Part model, mm, in its own coordinate system. Face numbers are marked on the shaded views. A direction names the side the tool comes from. Give positions to 0.01 mm unless a question says otherwise; leave off trailing zeros. Order: outer loops, then holes, each group sorted by start corner. A loop starts at its lowest first (then second) coordinate and runs counter-clockwise, first axis right, second up.
1. Slice it at D-D on z = 36. List the corners of the cut face in (x, y), and give its area (3 significant figures).
2. Which spindle directions (+Z, -Z, +X, -X, +Y, -Y) get a long thin tool onto all of the face, cutting with end or side? Do the marked faces 1 and 2. Say none if no direction does.
3. Slice it at B-B on y = 0. List the corners of the cut face in (x, z).
4. Probe line 1 (Y direction, x = -15.5, z = 20); line 2 (X direction, y = -15.5, z = 15.7). List the from-to ranges inside material, lowest first.
5. Slice it at A-A on z = 7.5. List the corners of the cut face in (x, y), and give its area (3 significant figures).
6. Drop flat-ended pins along their axis: pin 1 Ø1.5 at (x, y) = (15.5, 15.5) entering from +Z; pin 2 Ø10 at (x, y) = (-11, 15) entering from +Z; pin 3 Ø2.5 at (x, y) = (15.5, -15) entering from -Z; pin 4 Ø2.5 at (y, z) = (20, 6) entering from +X. Give the stop position or say it passes through.
7. Slice it at C-C on x = 0. List the corners of the cut face in (y, z), and give its area (3 significant figures).
Autodesk Inventor part; units mm, degrees
ref_plane "YZ Plane" through (0, 0, 0) normal (1, 0, 0) x (0, 1, 0)
ref_plane "XZ Plane" through (0, 0, 0) normal (0, 1, 0) x (-1, 0, 0)
ref_plane "XY Plane" through (0, 0, 0) normal (0, 0, 1) x (1, 0, 0)
sketch "Sketch1" plane through (0, 0, 0) normal (0, 0, 1) x (1, 0, 0)
  line L0 (-18.15, 21.15) -> (18.15, 21.15)
  line L1 (21.15, 18.15) -> (21.15, -18.15)
  line L2 (18.15, -21.15) -> (-18.15, -21.15)
  line L3 (-21.15, -18.15) -> (-21.15, 18.15)
  line L4 (-21.15, 21.15) -> (21.15, -21.15) construction
  line L5 (21.15, 21.15) -> (-21.15, -21.15) construction
  line L6 (18.15, 21.15) -> (21.15, 18.15)
  line L7 (-18.15, 21.15) -> (-21.15, 18.15)
  line L8 (-21.15, -18.15) -> (-18.15, -21.15)
  line L9 (18.15, -21.15) -> (21.15, -18.15)
  line L10 (-15.5, 15.5) -> (15.5, 15.5) construction
  line L11 (15.5, 15.5) -> (15.5, -15.5) construction
  line L12 (15.5, -15.5) -> (-15.5, -15.5) construction
  line L13 (-15.5, -15.5) -> (-15.5, 15.5) construction
  line L14 (-15.5, 15.5) -> (15.5, -15.5) construction
  line L15 (15.5, 15.5) -> (-15.5, -15.5) construction
  circle A0 centre (-15.5, 15.5) radius 1.5
  circle A1 centre (15.5, 15.5) radius 1.5
  circle A2 centre (15.5, -15.5) radius 1.5
  circle A3 centre (-15.5, -15.5) radius 1.5
  point P0 (0, 0)
  dimension "d0" = 42.3
  dimension "d1" = 42.3
  dimension "d2" = 3
  dimension "d3" = 3
  dimension "d4" = 3
  dimension "d5" = 3
  dimension "d6" = 3
  dimension "d7" = 3
  dimension "d8" = 3
  dimension "d9" = 3
  dimension "d10" = 31
  dimension "d11" = 31
  dimension "d12" = 3
  dimension "d13" = 3
  dimension "d14" = 3
  dimension "d15" = 3
extrude "Extrusion1" add sketch "Sketch1" along normal blind 10
sketch "Sketch2" plane through (0, 0, 10) normal (0, 0, 1) x (1, 0, 0)
  line L0 (-18.15, 21.15) -> (18.15, 21.15)
  line L1 (21.15, 18.15) -> (21.15, -18.15)
  line L2 (18.15, -21.15) -> (-18.15, -21.15)
  line L3 (-21.15, -18.15) -> (-21.15, 18.15)
  line L4 (-21.15, 21.15) -> (21.15, -21.15) construction
  line L5 (21.15, 21.15) -> (-21.15, -21.15) construction
  line L6 (-18.15, 21.15) -> (-21.15, 18.15)
  line L7 (-21.15, -18.15) -> (-18.15, -21.15)
  line L8 (21.15, -18.15) -> (18.15, -21.15)
  line L9 (18.15, 21.15) -> (21.15, 18.15)
  point P0 (0, 0)
  dimension "d18" = 42.3
  dimension "d19" = 42.3
  dimension "d20" = 3
  dimension "d21" = 3
  dimension "d22" = 3
  dimension "d23" = 3
  dimension "d24" = 3
  dimension "d25" = 3
  dimension "d26" = 3
  dimension "d27" = 3
extrude "Extrusion2" add sketch "Sketch2" along normal blind 3.5
sketch "Sketch3" plane through (0, 0, 13.5) normal (0, 0, 1) x (1, 0, 0)
  line L0 (-18.15, 21.15) -> (18.15, 21.15)
  line L1 (21.15, 18.15) -> (21.15, -18.15)
  line L2 (18.15, -21.15) -> (-18.15, -21.15)
  line L3 (-21.15, -18.15) -> (-21.15, 18.15)
  line L4 (-21.15, 21.15) -> (21.15, -21.15) construction
  line L5 (21.15, 21.15) -> (-21.15, -21.15) construction
  line L6 (-18.15, 21.15) -> (-21.15, 18.15)
  line L7 (-21.15, -18.15) -> (-18.15, -21.15)
  line L8 (21.15, -18.15) -> (18.15, -21.15)
  line L9 (18.15, 21.15) -> (21.15, 18.15)
  line L10 (-15.5, 15.5) -> (15.5, 15.5) construction
  line L11 (15.5, 15.5) -> (15.5, -15.5) construction
  line L12 (15.5, -15.5) -> (-15.5, -15.5) construction
  line L13 (-15.5, -15.5) -> (-15.5, 15.5) construction
  line L14 (-15.5, 15.5) -> (15.5, -15.5) construction
  line L15 (15.5, 15.5) -> (-15.5, -15.5) construction
  circle A0 centre (-15.5, 15.5) radius 0.5
  circle A1 centre (-15.5, -15.5) radius 0.5
  circle A2 centre (15.5, -15.5) radius 0.5
  circle A3 centre (15.5, 15.5) radius 0.5
  point P0 (0, 0)
  dimension "d30" = 42.3
  dimension "d31" = 42.3
  dimension "d32" = 3
  dimension "d33" = 3
  dimension "d34" = 3
  dimension "d35" = 3
  dimension "d36" = 3
  dimension "d37" = 3
  dimension "d38" = 3
  dimension "d39" = 3
  dimension "d40" = 31
  dimension "d41" = 31
  dimension "d42" = 1
  dimension "d43" = 1
  dimension "d44" = 1
  dimension "d45" = 1
extrude "Extrusion3" add sketch "Sketch3" along normal blind 10
sketch "Sketch4" plane through (0, 0, 23.5) normal (0, 0, 1) x (1, 0, 0)
  circle A0 centre (0, 0) radius 11
  dimension "d48" = 22
extrude "Extrusion4" add sketch "Sketch4" along normal blind 2
chamfer "Chamfer1" distance 0.5 angle 45 1 edges at (-11, 0, 25.5)
sketch "Sketch5" plane through (0, 0, 25.5) normal (0, 0, 1) x (1, 0, 0)
  circle A0 centre (0, 0) radius 10.5
  circle A1 centre (0, 0) radius 2.5
  dimension "d54" = 5
extrude "Extrusion5" add sketch "Sketch5" along normal blind 22 contours A1
sketch "Sketch6" plane through (-18.15, 21.15, 0) normal (0, 1, 0) x (1, 0, 0)
  line L0 (0, 0) -> (36.3, 0)
  line L1 (13.15, -1) -> (23.15, -1)
  line L2 (23.15, -1) -> (23.15, -9)
  line L3 (23.15, -9) -> (13.15, -9)
  line L4 (13.15, -9) -> (13.15, -1)
  line L5 (13.15, -1) -> (23.15, -9) construction
  line L6 (23.15, -1) -> (13.15, -9) construction
  point P0 (18.15, 0)
  point P1 (18.15, -5)
  dimension "d57" = 10
  dimension "d58" = 8
  dimension "d59" = 0
  dimension "d60" = 5
extrude "Extrusion6" cut sketch "Sketch6" against normal blind 5
sketch "Sketch7" plane through (0, 0, 47.5) normal (0, 0, 1) x (1, 0, 0)
  circle A0 centre (0, 0) radius 2.5
  arc A1 (1.8231, 1.7107) -> (-1.8197, 1.7142) centre (0, 0) ccw
  line L0 (-1.8197, 1.7142) -> (1.8231, 1.7107)
  dimension "d63" = 3.6428
extrude "Extrusion7" cut sketch "Sketch7" against normal blind 10 contours L0 A0 picked at (0.4606, 1.8369)
sketch "Esboço10" plane through (0, 0, 23.5) normal (0, 0, 1) x (1, 0, 0)
  circle A0 centre (15.5, 15.5) radius 0.5
  circle A1 centre (15.5, -15.5) radius 0.5
  circle A2 centre (-15.5, -15.5) radius 0.5
  circle A3 centre (-15.5, 15.5) radius 0.5
hole "Furo1" at (-15.5, 15.5, 23.5) at (15.5, 15.5, 23.5) at (15.5, -15.5, 23.5) at (-15.5, -15.5, 23.5) direction (0, 0, -1) diameter 2.459 depth 6 tip angle 118
sketch "Sketch9" plane through (0, 0, 0) normal (0, 0, -1) x (-1, 0, 0)
  circle A0 centre (0, 0) radius 2.5
  dimension "d68" = 5
equation "\"d3\" = d2"
equation "\"d4\" = d2"
equation "\"d5\" = d4"
equation "\"d6\" = d2"
equation "\"d7\" = d6"
equation "\"d8\" = d2"
equation "\"d9\" = d8"
equation "\"d21\" = d20"
equation "\"d23\" = d22"
equation "\"d24\" = d22"
equation "\"d25\" = d24"
equation "\"d26\" = d22"
equation "\"d27\" = d26"
equation "\"d33\" = d32"
equation "\"d34\" = d32"
equation "\"d35\" = d34"
equation "\"d36\" = d32"
equation "\"d37\" = d36"
equation "\"d38\" = d32"
equation "\"d39\" = d38"
properties part number "KTC-5017-010" material "Steel, Carbon"
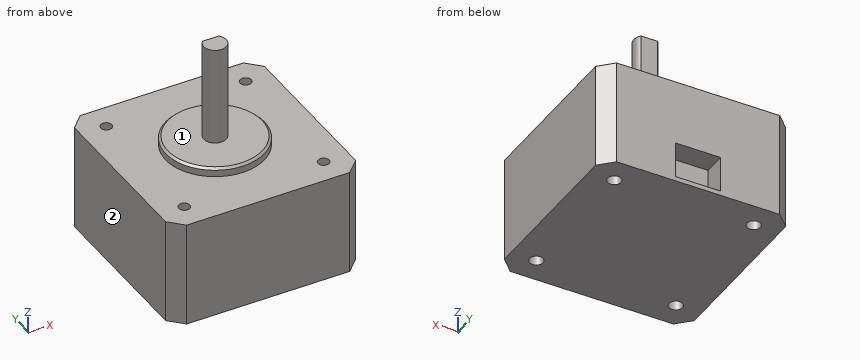
Data:
1. outline: circle Ø5 at (0, 0)
1. area: 19.6 mm2
2. face 1: +Z
2. face 2: +Z, -Z, -X, +Y, -Y
3. outline: (-21.15, 0) - (21.15, 0) - (21.15, 23.5) - (11, 23.5) - (11, 25) - (10.5, 25.5) - (2.5, 25.5) - (2.5, 47.5) - (-2.5, 47.5) - (-2.5, 25.5) - (-10.5, 25.5) - (-11, 25) - (-11, 23.5) - (-21.15, 23.5) - close
4. line 1: y = -21.15 to -16.73, -14.27 to 14.27, 16.73 to 21.15
4. line 2: x = -21.15 to -16, -15 to 15, 16 to 21.15
5. outline: (-21.15, -18.15) - (-18.15, -21.15) - (18.15, -21.15) - (21.15, -18.15) - (21.15, 18.15) - (18.15, 21.15) - (5, 21.15) - (5, 16.15) - (-5, 16.15) - (-5, 21.15) - (-18.15, 21.15) - (-21.15, 18.15) - close; hole circle Ø3 at (-15.5, -15.5); hole circle Ø3 at (-15.5, 15.5); hole circle Ø3 at (15.5, -15.5); hole circle Ø3 at (15.5, 15.5)
5. area: 1,690 mm2
6. pin 1: stops at z = 17.21
6. pin 2: stops at z = 23.5
6. pin 3: stops at z = 0
6. pin 4: stops at x = 20.55
7. outline: (-21.15, 0) - (21.15, 0) - (21.15, 1) - (16.15, 1) - (16.15, 9) - (21.15, 9) - (21.15, 23.5) - (11, 23.5) - (11, 25) - (10.5, 25.5) - (2.5, 25.5) - (2.5, 37.5) - (1.71, 37.5) - (1.71, 47.5) - (-2.5, 47.5) - (-2.5, 25.5) - (-10.5, 25.5) - (-11, 25) - (-11, 23.5) - (-21.15, 23.5) - close
7. area: 1,100 mm2
